Build history of the part. All positions in model axes, mm. A direction names the side the tool comes from. Round coordinates to 2 decimals unless told otherwise and drop trailing zeros. Loops run counter-clockwise (first coordinate to the right, second up) from the corner with the lowest first, then second, coordinate; pieces in that order, holes last. Notation, with made-up numbers: (-5, 16) - (12, 16) arc R15 cw to (12, 32) - close; hole circle Ø2 at (-13, 49.25). An arc over 180 degrees is marked (long way). Use a Markdown table: item, result.
from build123d import *

# Parameters (mm, degrees)
SKETCH2_R           = 3.5
SKETCH2_R_2         = 2.6
BOSS_EXTRUDE1_DEPTH = 14.6
SKETCH4_W           = 39.254699086
SKETCH4_H           = 35.178673269
CUT_EXTRUDE1_DEPTH  = 0.1
BOSS_EXTRUDE5_DEPTH = 14.5


with BuildPart() as part:
    # Sketch2 → Boss-Extrude1 (new body)
    # profile 1 of 2: a face of its own
    with BuildSketch(Plane(origin=(0, 0, 0), x_dir=(1, 0, 0), z_dir=(0, 1, 0))):
        with BuildLine():
            Line((-3.5, 17.5), (-3.5, 0))
            ThreePointArc((-3.5, 0), (0, 3.5), (3.5, 0))
            Line((3.5, 0), (17.206279241, 0))
            ThreePointArc((17.206279241, 0), (10.055441712, 12.539014932), (-3.5, 17.5))
        make_face()
    # profile 2 of 2: a face of its own
    with BuildSketch(Plane(origin=(0, 0, 0), x_dir=(1, 0, 0), z_dir=(0, 1, 0))):
        Circle(SKETCH2_R)
        with Locations(Location((0, 0, 0), (0, 0, 270))):
            Circle(SKETCH2_R_2, mode=Mode.SUBTRACT)
    extrude(amount=BOSS_EXTRUDE1_DEPTH)

    # Sketch4 → Cut-Extrude1 (cut)
    with BuildSketch(Plane(origin=(0, 14.6, 0), x_dir=(1, 0, 0), z_dir=(0, 1, 0))):
        with Locations((10.965886391, 4.797703191)):
            Rectangle(SKETCH4_W, SKETCH4_H)
    extrude(amount=-CUT_EXTRUDE1_DEPTH, mode=Mode.SUBTRACT)

    # Sketch7 → Boss-Extrude5 (add)
    with BuildSketch(Plane(origin=(0, 0, 0), x_dir=(-1, 0, 0), z_dir=(0, -1, 0))):
        with BuildLine():
            ThreePointArc((-11.881011918, -3.5), (-11.5942237, -3.409576022), (-11.411165608, -3.171010072))
            Line((-11.411165608, -3.171010072), (-10.257012329, 0))
            Line((-10.257012329, 0), (-13.505011507, 0))
            Line((-13.505011507, 0), (-17.206279241, 0))
            Line((-17.206279241, 0), (-13.505011507, -3.5))
            Line((-13.505011507, -3.5), (-11.881011918, -3.5))
        make_face()
    extrude(amount=-BOSS_EXTRUDE5_DEPTH)


solid = part.part
Q1. Probe line 1 (X direction, y = 1.5, z = -0.5); line 2 (X direction, y = 10.75, z = -1); line 3 (Z direction, x = 0, y = 6). List the from-to ranges inside material, lowest first.
Results found:
| item | result |
|---|---|
| line 1 | x = -3.5 to -2.55, 2.55 to 17.12 |
| line 2 | x = -3.5 to -2.4, 2.4 to 17.01 |
| line 3 | z = -17.21 to -2.6, 2.6 to 3.5 |
Q2. Cut at D-D, the plane z = -10.75. List the corners of the cut face in (x, y), plus the area to 3 significant figures.
Results found:
| item | result |
|---|---|
| outline | (-3.5, 0) - (11.93, 0) - (11.93, 14.5) - (-3.5, 14.5) - close |
| area | 224 mm2 |
Q3. Cut at A-A, the plane y = 4.75. List the corners of the cut face in (x, z).
Results found:
| item | result |
|---|---|
| outline | (-3.5, -17.5) arc R21 ccw to (17.21, 0) - (13.51, 3.5) - (11.88, 3.5) arc R0.5 ccw to (11.41, 3.17) - (10.26, 0) - (3.5, 0) arc R3.5 ccw to (-3.5, 0) - close; hole circle Ø5.2 at (0, 0) |
Q4. Which spindle directions (+Z, -Z, +X, -X, +Y, -Y) get a long thin tool onto all of the face, cutting with end or side? Do faces 1 (the face through (7, 7, 0)), 2 (the face through (13, 7, 3.5)). Say none if no direction does.
Results found:
| item | result |
|---|---|
| face 1 | +Z, +Y, -Y |
| face 2 | +Z, +X, -X, +Y, -Y |
Q5. Cut at B-B, the plane x = 0. List the corners of the cut face in (y, z), plus the area to 3 significant figures.
Results found:
| item | result |
|---|---|
| outline | (0, -17.21) - (14.5, -17.21) - (14.5, -2.6) - (0, -2.6) - close; (0, 2.6) - (14.5, 2.6) - (14.5, 3.5) - (0, 3.5) - close |
| area | 225 mm2 |
Q6. Pull direction X, two halves, no side cores. Call faces 3 (the face through (5, 14.5, -7)), 4 (the face through (0.78, 7.15, 2.48)), 5 (the face through (15.382, 7.148, 1.725)): pulls with the +X half, pulls with the -X half, needs draft (parallel to the pull), parting line crosses it, or undercut.
Results found:
| item | result |
|---|---|
| face 3 | needs draft |
| face 4 | undercut |
| face 5 | pulls with the +X half |
Q7. Cut at C-C, the plane z = 0.5. List the corners of the cut face in (x, y), plus the area to 3 significant figures.
Results found:
| item | result |
|---|---|
| outline | (-3.46, 0) - (-2.55, 0) - (-2.55, 14.5) - (-3.46, 14.5) - close; (2.55, 0) - (3.46, 0) - (3.46, 14.5) - (2.55, 14.5) - close; (10.44, 0) - (16.68, 0) - (16.68, 14.5) - (10.44, 14.5) - close |
| area | 117 mm2 |
Q8. Drop flat-ended pins along their axis: pin 1 (1.5 mm diameter, centred on y = 12.5, z = -6, fed in from +X); pin 2 (5 mm diameter, centred on x = 4.5, y = 10.5, fed in from +Z); pin 3 (6 mm diameter, centred on y = 12.5, z = -12.5, fed in from +X); pin 4 (4 mm diameter, centred on x = 0, z = 0, fed in from -Y). Give the stop position or say it passes through.
Results found:
| item | result |
|---|---|
| pin 1 | stops at x = 15.59 |
| pin 2 | stops at z = 2.87 |
| pin 3 | stops at x = 12.99 |
| pin 4 | passes through |
